from build123d import *

# Parameters (mm, degrees)
F2_W      = 16
F2_H      = 12.7785220167
F3_DEPTH  = 46.001
F4_W      = 23.5
F4_H      = 13.4564294844
F5_DEPTH  = 3.5
F6_W      = 23.5
F6_H      = 13.0310004231
F7_DEPTH  = 3.8
F8_R      = 10.75
F9_DEPTH  = 25
F11_W     = 31.7701289256
F11_H     = 9.9966360929
F12_DEPTH = 46.001
F14_R     = 1


with BuildPart() as f1:
    # F0 (on Front) → F1 (revolve)
    with BuildSketch(Plane.XZ):
        Polygon((-15.5, 0), (-13, 0), (-13, 3.8), (-10.5, 3.8), (-10.5, 42.5), (-13, 42.5), (-13, 46), (-15.5, 46), (-15.5, 42.5), (-13, 40), (-13, 6), (-15.5, 3.8), align=None)
    revolve(axis=Axis((0, 0, 24.8965322971), (0, 0, 1)))

    # F2 (on face) → F3 (cut, through all)
    with BuildSketch(Plane.XY.offset(46)):
        with Locations((0, 11.7036290467)):
            Rectangle(F2_W, F2_H)
    extrude(amount=-F3_DEPTH, mode=Mode.SUBTRACT)

    # F4 (on face) → F5 (cut, through all)
    with BuildSketch(Plane.XY.offset(46)):
        with Locations((0, 10.8011863194)):
            Rectangle(F4_W, F4_H)
    extrude(amount=-F5_DEPTH, mode=Mode.SUBTRACT)

    # F6 (on face) → F7 (cut, through all)
    with BuildSketch(Plane(origin=(0, 0, 0), x_dir=(1, 0, 0), z_dir=(0, 0, -1))):
        with Locations((0, -9.3560743844)):
            Rectangle(F6_W, F6_H)
    extrude(amount=-F7_DEPTH, mode=Mode.SUBTRACT)

    # F8 (on Front) → F9 (cut)
    with BuildSketch(Plane.XZ):
        with Locations((0, 29.25)):
            Circle(F8_R)
    extrude(amount=F9_DEPTH, mode=Mode.SUBTRACT)

    # F11 (on Top) → F12 (cut, through all)
    with BuildSketch(Plane.XY):
        with Locations((0.0608135015, 15.107101356)):
            Rectangle(F11_W, F11_H)
    extrude(amount=F12_DEPTH, mode=Mode.SUBTRACT)

    # F14
    f14_edges = [f1.edges().sort_by_distance(p)[0] for p in [
        (0.039521, -10.499926, 18.500073),
    ]]
    fillet(f14_edges, radius=F14_R)


solid = f1.part
Geometry check sheet. Reference: the model listing, model coordinates, mm. A direction names the side the tool comes from. Give positions to 0.01 mm unless a question says otherwise; leave off trailing zeros. Order: outer loops, then holes, each group sorted by start corner. A loop starts at its lowest first (then second) coordinate and runs counter-clockwise, first axis right, second up.
1) Cross-section at C-C (z = 43). Record the boundary of the cut face in (x, y), then the cut area to 3 significant figures.
Results are:
outline: (-11.75, 5.56) - (-11.75, 10.11) arc R15.5 ccw (long way) to (11.75, 10.11) - (11.75, 5.56) arc R13 cw (long way) to start
area: 154 mm2
2) Cross-section at D-D (z = 15). Record the boundary of the cut face in (x, y), then the cut area to 3 significant figures.
Results are:
outline: (-8.17, 10.11) arc R13 ccw (long way) to (8.17, 10.11) - (8, 10.11) - (8, 6.8) arc R10.5 cw (long way) to (-8, 6.8) - (-8, 10.11) - close
area: 140 mm2
3) Gauge pin test, flat ends, axial feed: pin 1 (2.5 mm diameter, centred on y = 9, z = 17.5, fed in from -X); pin 2 (7 mm diameter, centred on x = 3, y = 2.5, fed in from -Z); pin 3 (5 mm diameter, centred on y = 0.5, z = 29.5, fed in from -X); pin 4 (3 mm diameter, centred on y = 8.5, z = 1.5, fed in from +X). Record the tip position at first contact, or that the pin passes through.
Results are:
pin 1: stops at x = -10.44
pin 2: passes through
pin 3: stops at x = -13
pin 4: stops at x = 13.83
4) Material ranges on probe 1 along X at (y, z) = (0, 18); probe 2 along X at (y, z) = (0, 43.8); probe 3 along Y at (x, z) = (0, 1.05), recorded low to high.
Results are:
probe 1: x = -13 to -10.5, 10.5 to 13
probe 2: x = -15.5 to -13, 13 to 15.5
probe 3: y = -15.5 to -13
5) Draft check along Z on faces 1 (the flat face through (8, 8, 23)), 2 (the cylindrical face through (7.49, -8.4, 36.96)), 3 (the flat face through (0.1, -13.2, 0)), 4 (the conical face through (-0.45, -13.11, 40.12)). Enter one of: released by +Z, released by -Z, zero draft, split by the parting line, or undercut.
Results are:
face 1: zero draft
face 2: undercut
face 3: released by -Z
face 4: undercut
6) Cross-section at B-B (y = -10). Give the number of separate pieces and of enclosed holes in the cut face, then the cut area to 3 significant figures.
Results are:
separate pieces: 4
enclosed holes: 0
area: 281 mm2
7) Cross-section at A-A (z = 35.5). Record the boundary of the cut face in (x, y), then the cut area to 3 significant figures.
Results are:
outline: (-8.75, -9.62) - (-8.75, -5.81) arc R10.5 cw to (-8, 6.8) - (-8, 10.11) - (-8.17, 10.11) arc R13 ccw to start; (8, 6.8) arc R10.5 cw to (8.75, -5.81) - (8.75, -9.62) arc R13 ccw to (8.17, 10.11) - (8, 10.11) - close
area: 91.0 mm2
8) Tool access check on faces 5 (the flat face through (-8, 8, 23)), 6 (the flat face through (-11.75, 8, 44)), 7 (the cylindrical face through (-7.141, -10.863, 18.984)), 8 (the flat face through (11.75, 8, 2)), 9 (the cylindrical face through (0, -13, 2)). Record the directions out of +Z, -Z, +X, -X, +Y, -Y that give a thin tool (end or side, any length) a straight path to the whole face; none if there is none.
Results are:
face 5: +Z, -Z, +Y
face 6: +Z, +Y
face 7: none
face 8: -Z, +Y
face 9: -Z
